from build123d import *

# Parameters (mm, degrees)
F1_DEPTH = 50
F3_DEPTH = 15
F4_DEPTH = 15


with BuildPart() as f1:
    # F0 (on Top) → F1 (new body)
    with BuildSketch(Plane.XY):
        Polygon((0, 40), (0, 37), (10, 37), (10, 32), (0, 0), (15, 0), (15, 40), align=None)
    extrude(amount=F1_DEPTH)

    # F2 (on Right) → F3 (join)
    with BuildSketch(Plane.YZ):
        Polygon((40, -5), (40, 0), (0, 0), (0, -5), (15, -5), (15, -10), (25, -10), (25, -5), align=None)
    extrude(amount=F3_DEPTH)

    # F2 (on Right) → F4 (join)
    with BuildSketch(Plane.YZ):
        Polygon((40, -5), (40, 0), (0, 0), (0, -5), (15, -5), (15, -10), (25, -10), (25, -5), align=None)
    extrude(amount=-F4_DEPTH)


solid = f1.part
Can you work these out from the model? Positions are in its coordinate system, mm. A direction names the side the tool comes from. Give positions to 0.01 mm unless a question says otherwise; leave off trailing zeros. Loops run counter-clockwise (first coordinate to the right, second up) from the corner with the lowest first, then second, coordinate; pieces in that order, holes last. Notation, with made-up numbers: (55, 51) -> (76, 51) arc R20 ccw to (76, 71) -> close; hole circle Ø7 at (14.25, 77). An arc over 180 degrees is marked (long way). Return JSON: item names as keys, results as strings.
Q1. I need wall thicknesses on probe 1 along Z at (x, y) = (3, 34.5); probe 2 along Z at (x, y) = (-8.5, 20.5); probe 3 along X at (y, z) = (36.5, 41). Which ranges of each line are inside material? Lowest first, please.
Checks:
{"probe 1": "z = -5 to 0", "probe 2": "z = -10 to 0", "probe 3": "x = 10 to 15"}
Q2. We'd pull the mould along Y, two halves only. Please class faces 1 (the face through (0, 38, 25)), 2 (the face through (0, 25, -8)), 3 (the face through (7, 0, 23)), 4 (the face through (-5, 20, 0)): released by +Y, released by -Y, zero draft, split by the parting line, or undercut.
Checks:
{"face 1": "zero draft", "face 2": "released by +Y", "face 3": "released by -Y", "face 4": "undercut"}
Q3. I want a section at A-A, the plane x = 4.75. List the corners of the cut face in (y, z) for me, then the cut area to 3 significant figures.
Checks:
{"outline": "(0, -5) -> (15, -5) -> (15, -10) -> (25, -10) -> (25, -5) -> (40, -5) -> (40, 50) -> (37, 50) -> (37, 0) -> (15.2, 0) -> (15.2, 50) -> (0, 50) -> close", "area": "1,160 mm2"}
Q4. I want a section at B-B, the plane z = 27. List the corners of the cut face in (x, y) for me, then the cut area to 3 significant figures.
Checks:
{"outline": "(0, 0) -> (15, 0) -> (15, 40) -> (0, 40) -> (0, 37) -> (10, 37) -> (10, 32) -> close", "area": "390 mm2"}
Q5. On a 3-axis mill with a long thin cutter (end or side, diameter ignored), from which of +Z, -Z, +X, -X, +Y, -Y can I reach the whole of each face in a straight line? I mean faces 5 (the face through (0, 32, -5)), 6 (the face through (0, 15, -7)), 7 (the face through (5, 16, 25)). Say none if no direction works.
Checks:
{"face 5": "-Z, +X, -X, +Y", "face 6": "-Z, +X, -X, -Y", "face 7": "+Z, -X"}
Q6. I want a section at C-C, the plane y = 35. List the corners of the cut face in (x, z) for me.
Checks:
{"outline": "(-15, -5) -> (15, -5) -> (15, 50) -> (10, 50) -> (10, 0) -> (-15, 0) -> close"}
Q7. I want a section at D-D, the plane x = 9. List the corners of the cut face in (y, z) for me, then the cut area to 3 significant figures.
Checks:
{"outline": "(0, -5) -> (15, -5) -> (15, -10) -> (25, -10) -> (25, -5) -> (40, -5) -> (40, 50) -> (37, 50) -> (37, 0) -> (28.8, 0) -> (28.8, 50) -> (0, 50) -> close", "area": "1,840 mm2"}
Q8. For pin 1 Ø12 at (x, y) = (-1.5, 35.5) entering from -Z; pin 2 Ø2.5 at (y, z) = (34.5, 33) entering from -X; pin 3 Ø2.5 at (x, z) = (-3, -7) entering from +Y, each with a flat end and sliding along its axis, tell me the tip position at first contact or that it passes through.
Checks:
{"pin 1": "stops at z = -5", "pin 2": "stops at x = 10", "pin 3": "stops at y = 25"}
